CAD build for the part. Positions are in the model's coordinates, mm. Face numbers are marked on the shaded views. Give positions to 0.01 mm unless a question says otherwise; leave off trailing zeros. Order: outer loops, then holes, each group sorted by start corner. A loop starts at its lowest first (then second) coordinate and runs counter-clockwise, first axis right, second up. Notation, with made-up numbers: (32.25, 59) -> (81.25, 59) arc R32 ccw to (81.25, 87) -> close; hole circle Ø9 at (-2, 58). An arc over 180 degrees is marked (long way). Use one line per item in the form item = value. Start each with the question number.
1) Probe line 1 (Y direction, x = 0.75, z = 4.3); line 2 (X direction, y = -8.5, z = 4.8); line 3 (Y direction, x = -4, z = 1.1). List the from-to ranges inside material, lowest first.
2) Cut at B-B, the plane z = 2.55. Give the cut face in (x, y), and give its area (3 significant figures).
3) Cut at D-D, the plane y = -10. Give the cut face in (x, z), and give its area (3 significant figures).
4) Mould opens along X. For the marked faces 1, 2, 3 and 4 say: pulls with the +X half, pulls with the -X half, needs draft (parallel to the pull), parting line crosses it, or undercut.
5) Drop a flat-ended pin along its axis: P1, Ø4.5, axis at x = 0, y = -40, coming from the -Z side. Give the stop position or say it passes through.
6) Cut at C-C, the plane y = -38.5. Give the cut face in (x, z).
7) Cut at A-A, the plane x = 0. Give the cut face in (y, z), and give its area (3 significant figures).
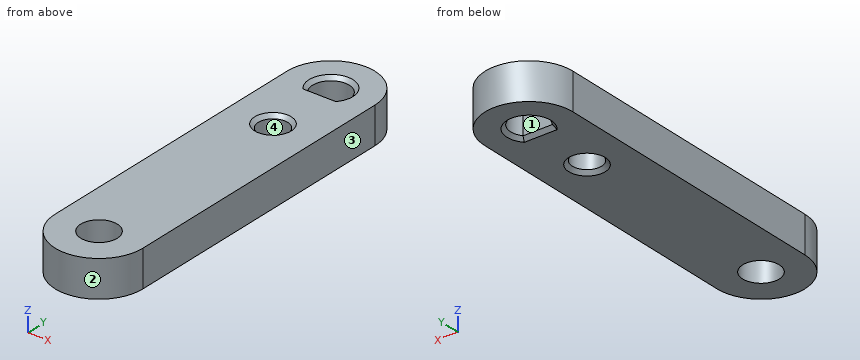
from build123d import *

# Parameters (mm, degrees)
SZKIC1_R                    = 2.5
SZKIC1_R_2                  = 2
DODANIE_WYCI_GNI_CIE1_DEPTH = 5
SFAZOWANIE1_SIZE            = 0.5


with BuildPart() as part:
    # Szkic1 → Dodanie-wyciągnięcie1 (new body)
    with BuildSketch(Plane.XY):
        with BuildLine():
            Line((6, -40), (6, 0))
            ThreePointArc((6, 0), (0, 6), (-6, 0))
            Line((-6, 0), (-6, -40))
            ThreePointArc((-6, -40), (0, -46), (6, -40))
        make_face()
        with Locations((0, -40)):
            Circle(SZKIC1_R, mode=Mode.SUBTRACT)
        with Locations((0, -10)):
            Circle(SZKIC1_R_2, mode=Mode.SUBTRACT)
        with BuildLine():
            Line((-2, -1.5), (2, -1.5))
            ThreePointArc((2, -1.5), (0, 2.5), (-2, -1.5))
        make_face(mode=Mode.SUBTRACT)
    extrude(amount=DODANIE_WYCI_GNI_CIE1_DEPTH)

    # Sfazowanie1
    sfazowanie1_edges = [part.edges().sort_by_distance(p)[0] for p in [
        (0, -1.5, 0),
        (0, 2.5, 0),
        (-2, -10, 0),
        (0, 2.5, 5),
        (0, -1.5, 5),
        (-2, -10, 5),
    ]]
    chamfer(sfazowanie1_edges, length=SFAZOWANIE1_SIZE)


solid = part.part
Result:
q1.line_1 = -45.95 to -42.38, -37.62 to -11.85, -8.15 to -1.5, 2.38 to 5.95
q1.line_2 = -6 to -1.74, 1.74 to 6
q1.line_3 = -44.47 to 4.47
q2.outline = (-6, -40) arc R6 ccw to (6, -40) -> (6, 0) arc R6 ccw to (-6, 0) -> close; hole circle Ø5 at (0, -40); hole circle Ø4 at (0, -10); hole (-2, -1.5) -> (2, -1.5) arc R2.5 ccw (long way) to start
q2.area = 544 mm²
q3.outline = (-6, 0) -> (-2.5, 0) -> (-2, 0.5) -> (-2, 4.5) -> (-2.5, 5) -> (-6, 5) -> close; (2, 0.5) -> (2.5, 0) -> (6, 0) -> (6, 5) -> (2.5, 5) -> (2, 4.5) -> close
q3.area = 39.5 mm²
q4.face_1 = undercut
q4.face_2 = parting line crosses it
q4.face_3 = pulls with the +X half
q4.face_4 = undercut
q5.P1 = through
q6.outline = (-6, 0) -> (-2, 0) -> (-2, 5) -> (-6, 5) -> close; (2, 0) -> (6, 0) -> (6, 5) -> (2, 5) -> close
q7.outline = (-46, 0) -> (-42.5, 0) -> (-42.5, 5) -> (-46, 5) -> close; (-37.5, 0) -> (-12.5, 0) -> (-12, 0.5) -> (-12, 4.5) -> (-12.5, 5) -> (-37.5, 5) -> close; (-8, 0.5) -> (-7.5, 0) -> (-2, 0) -> (-1.5, 0.5) -> (-1.5, 4.5) -> (-2, 5) -> (-7.5, 5) -> (-8, 4.5) -> close; (2.5, 0.5) -> (3, 0) -> (6, 0) -> (6, 5) -> (3, 5) -> (2.5, 4.5) -> close
q7.area = 194 mm²
